from build123d import *

# Parameters (mm, degrees)
F1_DEPTH = 10
F2_R     = 4.99999
F3_R     = 4.99999
F4_R     = 1
F5_R     = 1


# Not quite as in the source:
# - a fillet or chamfer is up to 0.001 mm smaller than in the source, because OpenCascade refuses the exact size


with BuildPart() as f1:
    # F0 (on Front) → F1 (new body)
    with BuildSketch(Plane.XZ):
        Polygon((0.5543106794, -10), (15.5543106794, -30), (45.5543106794, -30), (64.6686726809, 0), (45.5543106794, 30), (15.5543106794, 30), (0.5543106794, 10), (-64.4456893206, 10), (-64.4456893206, -10), align=None)
        with BuildLine():
            ThreePointArc((32.9945951312, 25.097839601), (47.7756292438, 17.8570035455), (54.8517478565, 2.9964106368))
            ThreePointArc((54.8517478565, 2.9964106368), (57.9982707821, -0.0333407521), (54.7851864872, -2.9924097466))
            ThreePointArc((54.7851864872, -2.9924097466), (47.5791639445, -17.4977896428), (32.9945951312, -24.542160399))
            ThreePointArc((32.9945951312, -24.542160399), (30, -27.722160399), (27.0054048688, -24.542160399))
            ThreePointArc((27.0054048688, -24.542160399), (12.4208360555, -17.4977896428), (5.2148135128, -2.9924097466))
            ThreePointArc((5.2148135128, -2.9924097466), (2.0017292179, -0.0333407521), (5.1482521435, 2.9964106368))
            ThreePointArc((5.1482521435, 2.9964106368), (12.2243707562, 17.8570035455), (27.0054048688, 25.097839601))
            ThreePointArc((27.0054048688, 25.097839601), (30, 28.277839601), (32.9945951312, 25.097839601))
        make_face(mode=Mode.SUBTRACT)
    extrude(amount=F1_DEPTH)

    # F2 (radius 5 in the source; OpenCascade refuses exactly that, so slightly less here)
    f2_edges = [f1.edges().sort_by_distance(p)[0] for p in [
        (-31.945689, -10, -10),
        (-31.945689, 0, -10),
    ]]
    fillet(f2_edges, radius=F2_R)

    # F3 (radius 5 in the source; OpenCascade refuses exactly that, so slightly less here)
    f3_edges = [f1.edges().sort_by_distance(p)[0] for p in [
        (-31.945689, 0, 10),
        (-31.945689, -10, 10),
    ]]
    fillet(f3_edges, radius=F3_R)

    # F4
    f4_edges = [f1.edges().sort_by_distance(p)[0] for p in [
        (8.054311, -10, 20),
        (30.554311, -10, 30),
        (55.111492, -10, 15),
        (55.111492, -10, -15),
        (30.554311, -10, -30),
        (8.054311, -10, -20),
    ]]
    fillet(f4_edges, radius=F4_R)

    # F5
    f5_edges = [f1.edges().sort_by_distance(p)[0] for p in [
        (30.554311, 0, 30),
        (55.111492, 0, 15),
        (55.111492, 0, -15),
        (30.554311, 0, -30),
        (8.054311, 0, -20),
        (8.054311, 0, 20),
    ]]
    fillet(f5_edges, radius=F5_R)


solid = f1.part
Geometry check sheet. Reference: the model listing, model coordinates, mm. A direction names the side the tool comes from. Give positions to 0.01 mm unless a question says otherwise; leave off trailing zeros. Order: outer loops, then holes, each group sorted by start corner. A loop starts at its lowest first (then second) coordinate and runs counter-clockwise, first axis right, second up. Notation, with made-up numbers: M -20,-8.75 L -9,-8.75 A11 ccw -9,11.25 Z; hole C -27,54 d7. An arc over 180 degrees is marked long. Use a Markdown table: item, result.
Item 1: Depth check by flat-ended pin: P1, Ø3, axis at x = -12, y = -2.5, coming from the +Z side; P2, Ø3, axis at y = -7.5, z = 21, coming from the +X side; P3, Ø6, axis at x = 10, y = -8, coming from the -Z side. Enter the tip coordinate at first touch or a pass-through.
Answers follow:
| item | result |
|---|---|
| P1 | stops at z = 9.9 |
| P2 | stops at x = 52.24 |
| P3 | stops at z = -26.59 |
Item 2: Section check A-A (x = 30). Record the cut outline in (y, z).
Answers follow:
| item | result |
|---|---|
| outline | M -10,-29 A1 ccw -9,-30 L -1,-30 A1 ccw 0,-29 L 0,-27.72 L -10,-27.72 Z; M -10,28.28 L 0,28.28 L 0,29 A1 ccw -1,30 L -9,30 A1 ccw -10,29 Z |
Item 3: Material ranges on line 1 along X through (y, z) = (-5, 5); line 2 along X through (y, z) = (-9, 18); line 3 along Z through (x, y) = (26.5, -2), recorded low to high.
Answers follow:
| item | result |
|---|---|
| line 1 | x = -64.45 to 5.45, 54.55 to 61.48 |
| line 2 | x = 6.55 to 12.37, 47.63 to 53.2 |
| line 3 | z = -30 to -24.48, 25.03 to 30 |
Item 4: Section check B-B (y = -7.25). Record the cut outline in (x, z).
Answers follow:
| item | result |
|---|---|
| outline | M -64.45,-9.47 L 0.15,-9.47 L 15.55,-30 L 45.55,-30 L 64.67,0 L 45.55,30 L 15.55,30 L 0.15,9.47 L -64.45,9.47 Z; hole M 5.15,3 A3 ccw long 5.21,-2.99 A25 ccw 27.01,-24.54 A3 ccw long 32.99,-24.54 A25 ccw 54.79,-2.99 A3 ccw long 54.85,3 A25 ccw 32.99,25.1 A3 ccw long 27.01,25.1 A25 ccw Z |
Item 5: Draft check along X on faces 4 (the cylindrical face through (54.992, -0.285, -14.628)), 5 (the cylindrical face through (47.743, -4.93, -17.335)), 6 (the cylindrical face through (6.517, -9.715, 17.449)), 7 (the cylindrical face through (58, -5, 0)). Enter one of: +X half, -X half, draft (parallel to the pull), parting line (faces both ways), or undercut.
Answers follow:
| item | result |
|---|---|
| face 4 | +X half |
| face 5 | undercut |
| face 6 | -X half |
| face 7 | undercut |
Item 6: Tool access check on faces 1 (the cylindrical face through (-32, -2, 9)), 2 (the cylindrical face through (30.07, -4.93, -27.72)), 3 (the cylindrical face through (-31, -8, -9)). Record the directions out of +Z, -Z, +X, -X, +Y, -Y that give a thin tool (end or side, any length) a straight path to the whole face; none if there is none.
Answers follow:
| item | result |
|---|---|
| face 1 | +Z, -X, +Y |
| face 2 | +Y, -Y |
| face 3 | -Z, -X, -Y |
